from build123d import *

# Parameters (mm, degrees)
SKETCH1_W           = 3
SKETCH1_H           = 24
BOSS_EXTRUDE1_DEPTH = 38
SKETCH2_W           = 2
SKETCH2_H           = 13.483919992
BOSS_EXTRUDE2_DEPTH = 20
CHAMFER1_SIZE       = 20
SKETCH3_W           = 38
SKETCH3_H           = 3
BOSS_EXTRUDE3_DEPTH = 20
SKETCH4_R           = 1.75
CUT_EXTRUDE1_DEPTH  = 51.487622245
SKETCH5_W           = 28
SKETCH5_H           = 20
BOSS_EXTRUDE4_DEPTH = 8
CUT_EXTRUDE2_DEPTH  = 8
SKETCH7_W           = 4.299558672
SKETCH7_H           = 5.002260433
CUT_EXTRUDE3_DEPTH  = 15
CUT_EXTRUDE4_DEPTH  = 15
FILLET3_R           = 2.5
SKETCH9_W           = 3
SKETCH9_H           = 10
BOSS_EXTRUDE5_DEPTH = 7.5
CHAMFER2_SIZE       = 7.5
FILLET4_R           = 2.5
SKETCH11_R          = 2
CUT_EXTRUDE5_DEPTH  = 47.840153715


# Some blends are built 0.0001 mm under size
with BuildPart() as part:
    # Sketch1 → Boss-Extrude1 (new body)
    with BuildSketch(Plane(origin=(0, 0, 0), x_dir=(0, 0, -1), z_dir=(1, 0, 0))):
        with Locations((1.5, 12)):
            Rectangle(SKETCH1_W, SKETCH1_H)
    extrude(amount=BOSS_EXTRUDE1_DEPTH)

    # Sketch2 → Boss-Extrude2 (add)
    with BuildSketch(Plane.XY):
        with Locations((19, 6.741959996)):
            Rectangle(SKETCH2_W, SKETCH2_H)
    extrude(amount=BOSS_EXTRUDE2_DEPTH)

    # Chamfer1
    # the kernel refuses this chamfer: 20 mm, written as the material it takes off along each edge
    with BuildSketch(Plane(origin=(71.433659759, 13.483919992, 20), x_dir=(0, 0.027495876610586403, -0.9996219169112968), z_dir=(-1, 0, 0))) as chamfer1_piece_1_section:
        Polygon((CHAMFER1_SIZE * 0.999621916911, CHAMFER1_SIZE * 0.0274958766106), (-CHAMFER1_SIZE * 0.0274958766106, CHAMFER1_SIZE * 0.999621916911), (0, 0), align=None)
    chamfer1_piece_1 = extrude(amount=104.867319519, mode=Mode.PRIVATE)
    chamfer1_piece_1 = split(chamfer1_piece_1, bisect_by=Plane(origin=(19, 6.875836906, 0), z_dir=(0, 0, 1)), keep=Keep.TOP, mode=Mode.PRIVATE)
    add(chamfer1_piece_1, mode=Mode.SUBTRACT)

    # Sketch3 → Boss-Extrude3 (add)
    with BuildSketch(Plane(origin=(0, 0, -3), x_dir=(-1, 0, 0), z_dir=(0, 0, -1))):
        with Locations((-19, 1.5)):
            Rectangle(SKETCH3_W, SKETCH3_H)
    extrude(amount=BOSS_EXTRUDE3_DEPTH)

    # Sketch4 → Cut-Extrude1 (cut, through all)
    with BuildSketch(Plane.XZ):
        with Locations(Location((2.5, -13, 0), (0, 0, 270))):
            Circle(SKETCH4_R)
        with Locations(Location((35.5, -13, 0), (0, 0, 270))):
            Circle(SKETCH4_R)
    extrude(amount=-CUT_EXTRUDE1_DEPTH, mode=Mode.SUBTRACT)

    # Sketch5 → Boss-Extrude4 (add)
    with BuildSketch(Plane(origin=(0, 3, 0), x_dir=(1, 0, 0), z_dir=(0, 1, 0))):
        with Locations((19, 13)):
            Rectangle(SKETCH5_W, SKETCH5_H)
    extrude(amount=BOSS_EXTRUDE4_DEPTH)

    # Sketch6 → Cut-Extrude2 (cut)
    with BuildSketch(Plane.XZ):
        Polygon((11, -23), (27, -23), (27, -20), (30, -20), (30, -3), (8, -3), (8, -20), (11, -20), align=None)
    extrude(amount=-CUT_EXTRUDE2_DEPTH, mode=Mode.SUBTRACT)

    # Sketch7 → Cut-Extrude3 (cut)
    with BuildSketch(Plane(origin=(0, 0, -3), x_dir=(-1, 0, 0), z_dir=(0, 0, -1))):
        with Locations((-27.850220664, 2.501130217)):
            Rectangle(SKETCH7_W, SKETCH7_H)
        with Locations((-10.149779336, 2.501130217)):
            Rectangle(SKETCH7_W, SKETCH7_H)
    extrude(amount=-CUT_EXTRUDE3_DEPTH, mode=Mode.SUBTRACT)

    # Sketch8 → Cut-Extrude4 (cut)
    with BuildSketch(Plane.ZY.offset(-18)):
        Polygon((7.858304832, 5.62561516), (7.858304832, 0), (13.483919992, 0), align=None)
    extrude(amount=-CUT_EXTRUDE4_DEPTH, mode=Mode.SUBTRACT)

    # Fillet3
    fillet3_edges = [part.edges().sort_by_distance(p)[0] for p in [
        (38, 1.5, -23),
        (0, 1.5, -23),
        (5, 7, -3),
        (33, 7, -3),
        (5, 11, -13),
        (19, 11, -3),
        (33, 11, -13),
        (19, 11, -23),
    ]]
    fillet(fillet3_edges, radius=FILLET3_R)

    # Sketch9 → Boss-Extrude5 (add)
    with BuildSketch(Plane(origin=(0, 11, 0), x_dir=(1, 0, 0), z_dir=(0, 1, 0))):
        with Locations((12.5, 8)):
            Rectangle(SKETCH9_W, SKETCH9_H)
        with Locations((25.5, 8)):
            Rectangle(SKETCH9_W, SKETCH9_H)
    extrude(amount=BOSS_EXTRUDE5_DEPTH)

    # Chamfer2
    chamfer2_edges = [part.edges().sort_by_distance(p)[0] for p in [
        (12.5, 18.5, -13),
        (25.5, 18.5, -13),
    ]]
    chamfer(chamfer2_edges, length=CHAMFER2_SIZE - 0.0001)  # a hair under: the kernel refuses the full size

    # Fillet4
    fillet4_edges = [part.edges().sort_by_distance(p)[0] for p in [
        (38, 24, -1.5),
        (0, 24, -1.5),
    ]]
    fillet(fillet4_edges, radius=FILLET4_R)

    # Sketch11 → Cut-Extrude5 (cut, through all)
    with BuildSketch(Plane(origin=(33, 0, 0), x_dir=(0, 0, -1), z_dir=(1, 0, 0))):
        with Locations((8.74878855, 5.75)):
            Circle(SKETCH11_R)
    extrude(amount=-CUT_EXTRUDE5_DEPTH, mode=Mode.SUBTRACT)


solid = part.part
Work out the finished part from the listing and answer in its coordinate system (mm). A direction names the side the tool comes from. Give positions to 0.01 mm unless a question says otherwise; leave off trailing zeros. Loops run counter-clockwise (first coordinate to the right, second up) from the corner with the lowest first, then second, coordinate; pieces in that order, holes last. Notation, with made-up numbers: M 19,60 L 23,60 A27 cw 23,90 Z; hole C 65,88.5 d1. An arc over 180 degrees is marked long. Use CSV: the item, a comma, the result in double quotes.
1) Consider L1, parallel to X at y = 1.55, z = -13; L2, parallel to X at y = 7.75, z = -10; L3, parallel to X at y = 1.5, z = -4. Determine where each line is inside the solid, lowest interval first.
Answer:
L1,"0 to 0.75, 4.25 to 8, 30 to 33.75, 37.25 to 38"
L2,"5 to 8, 30 to 33"
L3,"0 to 8, 30 to 38"
2) Find section D-D on x = 10. Write down the section's boundary in (y, z).
Answer:
outline,"M 0,-23 L 8.5,-23 A2.5 ccw 11,-20.5 L 11,-5.5 A2.5 cw 13.5,-3 L 24,-3 L 24,0 L 5,0 L 5,-3 L 8,-3 L 8,-20 L 0,-20 Z"
3) Find section B-B on x = 21.5. Write down the section's boundary in (y, z), plus the area to 3 significant figures.
Answer:
outline,"M 0,-3 L 8,-3 L 8,-23 L 8.5,-23 A2.5 ccw 11,-20.5 L 11,-5.5 A2.5 cw 13.5,-3 L 24,-3 L 24,0 L 0,0 Z"
area,"132 mm^2"
4) Given P1, Ø1.5, axis at x = 14.5, z = -19, coming from the +Y side; P2, Ø5, axis at x = 25.5, y = 15.5, coming from the +Z side; P3, Ø4, axis at x = 2, z = -15.5, coming from the +Y side, each flat-ended and moving along its own axis, determine where each tip first touches the part or whether it passes through.
Answer:
P1,"y = 11"
P2,"z = 0"
P3,"y = 3"
5) Determine the mould class of faces 4 (the cylindrical face through (0.713, 23.248, -1.521)), 5 (the cylindrical face through (28.774, 11.752, -3.713)), 6 (the flat face through (27, 4, -22)), 7 (the cylindrical face through (37.287, 1.521, -22.248)) for opening direction X: released by +X, released by -X, zero draft, split by the parting line, or undercut.
Answer:
face 4,"released by -X"
face 5,"zero draft"
face 6,"undercut"
face 7,"released by +X"
6) Find section A-A on z = -8.5. Give the number of separate pieces and of enclosed holes in the cut face, plus the area to 3 significant figures.
Answer:
separate pieces,"3"
enclosed holes,"0"
area,"163 mm^2"
7) Which of the six approach directions +Z, -Z, +X, -X, +Y, -Y give full straight-line access (tool end or side, diameter ignored) to faces 1 (the cylindrical face through (4.248, 5.788, -3.713)), 2 (the flat face through (14, 14, -7)), 3 (the flat face through (12, 18.5, -4))?
Answer:
face 1,"-Z, -X, +Y"
face 2,"-Z, +Y"
face 3,"-Z, +X, -X, +Y"
